For this review, use the dimensioned drawing (mm, ordinates from the lowest corner) and the shaded views. A direction names the side the tool comes from. Round coordinates to 2 decimals unless told otherwise and drop trailing zeros. Write each loop counter-clockwise with the first axis right and the second up, starting at its lowest first coordinate (ties: lowest second). Pieces come first, ordered by that corner, then holes. Notation, with made-up numbers: (47.5, 35.25) -> (93.5, 35.25) arc R18 ccw to (93.5, 41.25) -> close; hole circle Ø8 at (62, 67.25). An arc over 180 degrees is marked (long way). Answer as CSV lines item,"result". Start each with the question number.
Item 1: Machinability: for the marked faces 1 and 2, which of the approach directions +Z, -Z, +X, -X, +Y, -Y give a long, thin tool a straight path to every point of the face, cutting with its end or side? Answer none if there is none.
Item 2: Mouldability with a two-part tool opening along X and no side actions: class the marked faces 3, 4 and 5 as +X half, -X half, draft (parallel to the pull), parting line (faces both ways), or undercut.
Item 3: For pin 1 Ø19 at (x, z) = (17.5, 32.5) entering from +Y (1 decimal); pin 2 Ø8 at (x, y) = (24.5, 36) entering from +Z (1 decimal), all flat-tipped, find the tip position at first contact; note any pin that passes through.
Item 4: Wall thickness on probe 1 along Y at (x, z) = (21, 35) (1 decimal); probe 2 along Y at (x, z) = (4, 4) (1 decimal): over which ranges is each line inside the solid? List them lowest first. Write a range as from..to.
Item 5: Take a section at B-B on z = 31.5. Give the boundary of the cut face in (x, y) (1 decimal), then the cut area to 3 significant figures.
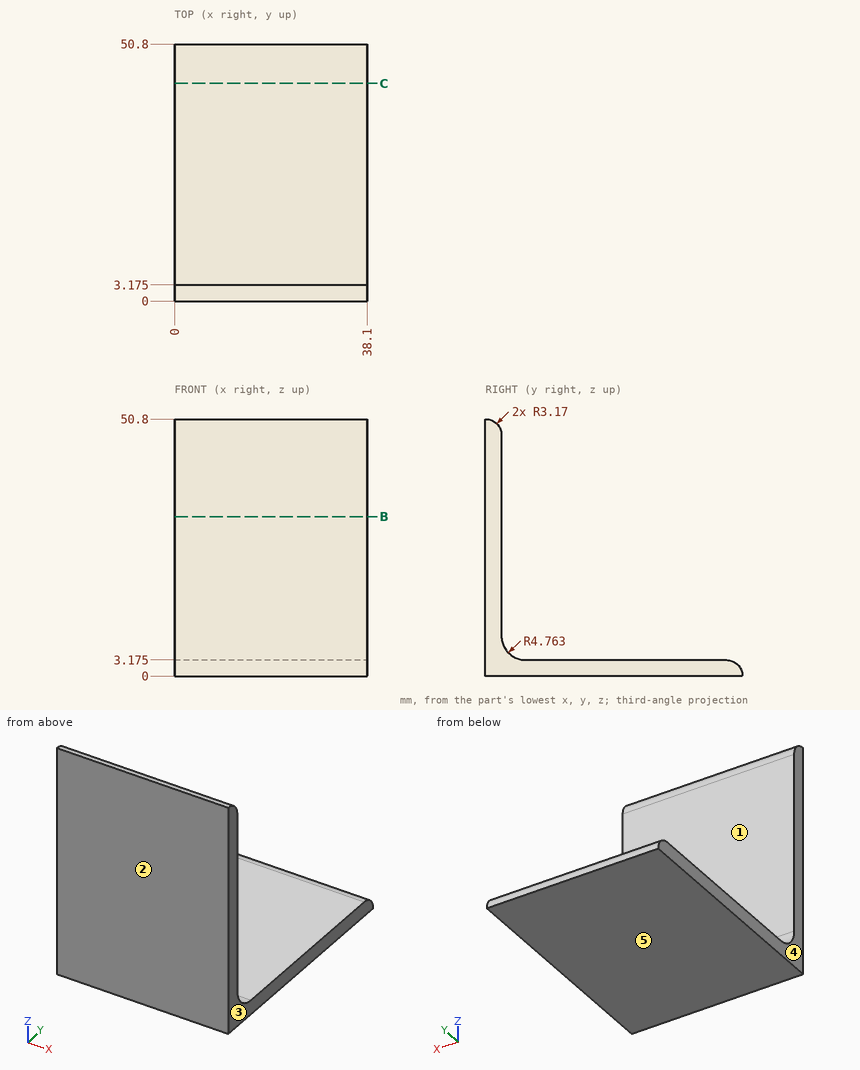
Output values:
1,face 1,"+Z, +X, -X, +Y"
1,face 2,"+Z, -Z, +X, -X, -Y"
2,face 3,"+X half"
2,face 4,"-X half"
2,face 5,"draft"
3,pin 1,"stops at y = 3.2"
3,pin 2,"stops at z = 3.2"
4,probe 1,"y = 0..3.2"
4,probe 2,"y = 0..5.3"
5,outline,"(0, 0) -> (38.1, 0) -> (38.1, 3.2) -> (0, 3.2) -> close"
5,area,"121 mm^2"
